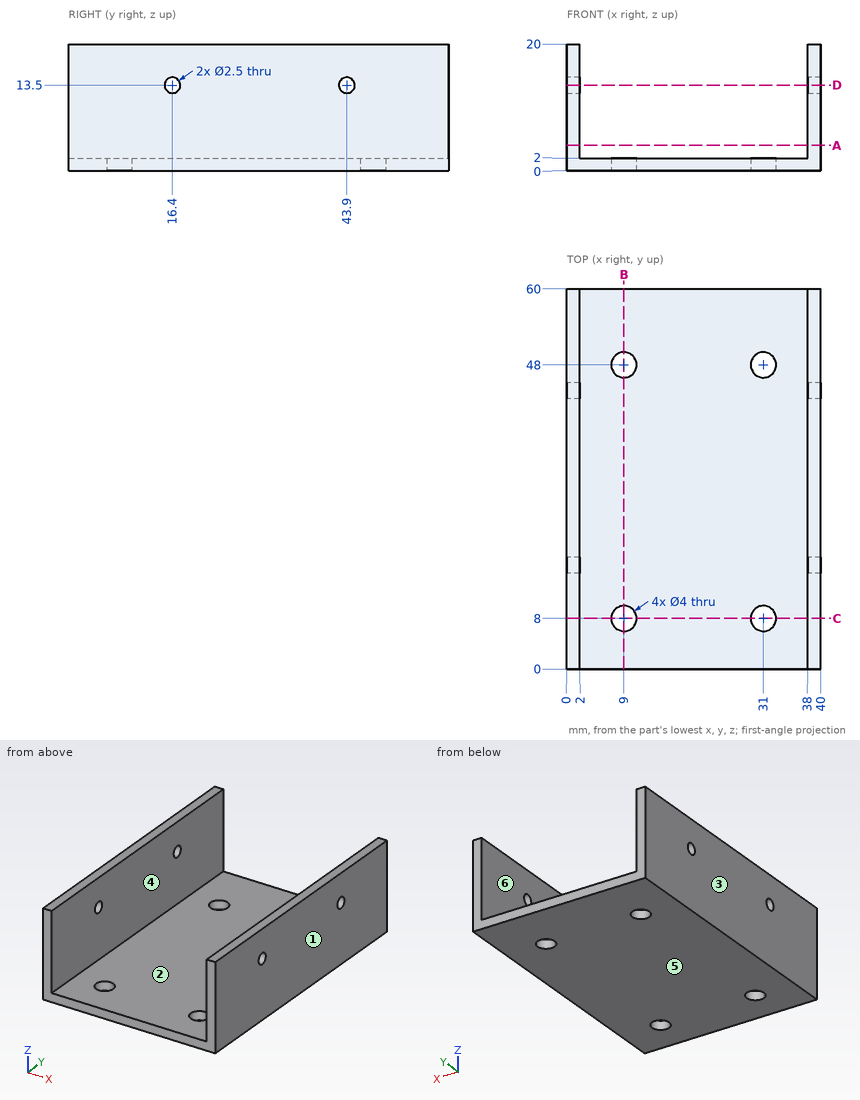
Print and shaded views of the part. All mm, measured from the part's lowest x, y and z. A direction names the side the tool comes from. Round coordinates to 2 decimals unless told otherwise and drop trailing zeros. Write each loop counter-clockwise with the first axis right and the second up, starting at its lowest first coordinate (ties: lowest second). Pieces come first, ordered by that corner, then holes. Notation, with made-up numbers: M 47,23 L 86,23 A22 ccw 86,46 Z; hole C 24.5,1.5 d2. An arc over 180 degrees is marked long. Use a Markdown table: item, result. Add a question column.
1. 3-axis set-ups, long thin cutter, end or side, ignore diameter. For the marked faces 1 and 2: which of +Z, -Z, +X, -X, +Y, -Y reach the whole face in a straight line?
2. Slice it at B-B on x = 9. Give the cut face in (y, z).
3. Slice it at D-D on z = 13.5. Give the cut face in (x, y), then the cut area to 3 significant figures.
4. Flat gauge pins, fed straight in: P1, Ø12, axis at x = 12, y = 51.5, coming from the -Z side; P2, Ø2, axis at y = 43.9, z = 13.5, coming from the -X side; P3, Ø11, axis at x = 25, y = 21, coming from the +Z side. Where does each tip first touch, or does it go through?
5. Drill centre lines: probe 1 along Y at (x, z) = (39, 13.5); probe 2 along Y at (x, z) = (9, 1.05); probe 3 along X at (y, z) = (17.5, 6). Where is each one in solid material? Low to high.
6. Pull direction X, two halves, no side cores. Call the marked faces 3, 4, 5 and 6: released by +X, released by -X, zero draft, split by the parting line, or undercut.
7. Slice it at A-A on z = 4. Give the cut face in (x, y), then the cut area to 3 significant figures.
8. Slice it at C-C on y = 8. Give the cut face in (x, z).
Reply:
| question | item | result |
|---|---|---|
| 1 | face 1 | +Z, -Z, +X, +Y, -Y |
| 1 | face 2 | +Z, +Y, -Y |
| 2 | outline | M 0,0 L 6,0 L 6,2 L 0,2 Z; M 10,0 L 46,0 L 46,2 L 10,2 Z; M 50,0 L 60,0 L 60,2 L 50,2 Z |
| 3 | outline | M 0,0 L 2,0 L 2,15.15 L 0,15.15 Z; M 0,17.65 L 2,17.65 L 2,42.65 L 0,42.65 Z; M 0,45.15 L 2,45.15 L 2,60 L 0,60 Z; M 38,0 L 40,0 L 40,15.15 L 38,15.15 Z; M 38,17.65 L 40,17.65 L 40,42.65 L 38,42.65 Z; M 38,45.15 L 40,45.15 L 40,60 L 38,60 Z |
| 3 | area | 220 mm^2 |
| 4 | P1 | stops at z = 0 |
| 4 | P2 | passes through |
| 4 | P3 | stops at z = 2 |
| 5 | probe 1 | y = 0 to 15.15, 17.65 to 42.65, 45.15 to 60 |
| 5 | probe 2 | y = 0 to 6, 10 to 46, 50 to 60 |
| 5 | probe 3 | x = 0 to 2, 38 to 40 |
| 6 | face 3 | released by -X |
| 6 | face 4 | undercut |
| 6 | face 5 | zero draft |
| 6 | face 6 | undercut |
| 7 | outline | M 0,0 L 2,0 L 2,60 L 0,60 Z; M 38,0 L 40,0 L 40,60 L 38,60 Z |
| 7 | area | 240 mm^2 |
| 8 | outline | M 0,0 L 7,0 L 7,2 L 2,2 L 2,20 L 0,20 Z; M 11,0 L 29,0 L 29,2 L 11,2 Z; M 33,0 L 40,0 L 40,20 L 38,20 L 38,2 L 33,2 Z |
